Input: part model. Units: mm. Frame: model coordinates. Give positions to 0.01 mm unless a question says otherwise; leave off trailing zeros. Order: outer loops, then holes, each group sorted by start corner. A loop starts at its lowest first (then second) coordinate and runs counter-clockwise, first axis right, second up. Notation, with made-up numbers: (78.5, 39.5) -> (118.5, 39.5) arc R23 ccw to (118.5, 64.5) -> close; hole circle Ø5 at (82, 85). An arc over 180 degrees is marked (long way). Use a Markdown table: item, result. Add a question column.
from build123d import *

# Parameters (mm, degrees)
SKETCH3_R           = 12.7
SKETCH4_R           = 12.7
BOSS_EXTRUDE3_DEPTH = 330.2
SKETCH5_R           = 12.7
BOSS_EXTRUDE4_DEPTH = 330.2
SKETCH7_W           = 12.7
SKETCH7_H           = 152.4
CUT_EXTRUDE2_DEPTH  = 6.35


with BuildPart() as part:
    # Sweep1: sweep along a path in Sketch2
    with BuildLine(Plane(origin=(0, 0, 0), x_dir=(0, 0, -1), z_dir=(1, 0, 0))) as sweep1_path:
        ThreePointArc((-64.833774642, 0), (-45.844401699, 45.844401699), (0, 64.833774642))
    # Sketch3 → Sweep1 (sweep)
    with BuildSketch(Plane(origin=(0, 0, 0), x_dir=(1, 0, 0), z_dir=(0, 1, 0))):
        with Locations((0, -64.833774642)):
            Circle(SKETCH3_R)
    sweep(path=sweep1_path.line)

    # Sketch4 → Boss-Extrude3 (add)
    with BuildSketch(Plane(origin=(0, 0, 0), x_dir=(-1, 0, 0), z_dir=(0, -1, 0))):
        with Locations(Location((0, -64.833774642, 0), (0, 0, 90))):
            Circle(SKETCH4_R)
    extrude(amount=BOSS_EXTRUDE3_DEPTH)

    # Sketch5 → Boss-Extrude4 (add)
    with BuildSketch(Plane(origin=(0, 0, 0), x_dir=(-1, 0, 0), z_dir=(0, 0, -1))):
        with Locations(Location((0, 64.833774642, 0), (0, 0, 90))):
            Circle(SKETCH5_R)
    extrude(amount=BOSS_EXTRUDE4_DEPTH)

    # Sketch7 → Cut-Extrude2 (cut)
    with BuildSketch(Plane(origin=(12.7, 0, 0), x_dir=(0, 0, -1), z_dir=(1, 0, 0))):
        with Locations((-63.5, -76.2)):
            Rectangle(SKETCH7_W, SKETCH7_H)
    extrude(amount=-CUT_EXTRUDE2_DEPTH, mode=Mode.SUBTRACT)


solid = part.part
Q1. First-contact query: pin 1 (6 mm diameter, centred on x = 8.5, y = -112, fed in from -Z); pin 2 (7 mm diameter, centred on x = 10.5, z = 64.5, fed in from +Y); pin 3 (12 mm diameter, centred on x = 7, z = -6, fed in from +Y). Flat tips, straight axial feed; report the tip coordinate or a pass-through.
Q2. Section query C-C (y = -99). Return loops of the section in (x, z).
Q3. Ray query, line 1 (Z direction, x = -0.25, y = -209); line 2 (Z direction, x = 9.5, y = -92); line 3 (Y direction, x = 9.25, z = -234). Return the intervals inside material, ascending.
Q4. Section query A-A (x = 0). Return loops of the section in (y, z).
Q5. Section query B-B (z = -253). Return loops of the section in (x, y), plus the area to 3 significant figures.
Q6. Draft query along Z for faces 1 (the flat face through (0, -330.2, 65)), 2 (the flat face through (0, 65, -330.2)), 3 (the flat face through (6.35, -75, 64)), 4 (the cylindrical face through (-12.398, -162.789, 67.587)). Return one class per face: +Z half, -Z half, draft (parallel to the pull), parting line (faces both ways), or undercut.
Solution:
| question | item | result |
|---|---|---|
| 1 | pin 1 | stops at z = 53.39 |
| 1 | pin 2 | stops at y = 41.59 |
| 1 | pin 3 | stops at y = 77.49 |
| 2 | outline | (6.35, 57.15) -> (6.35, 69.85) -> (11.67, 69.85) arc R12.7 ccw (long way) to (10.11, 57.15) -> close |
| 3 | line 1 | z = 52.14 to 77.53 |
| 3 | line 2 | z = 56.41 to 57.15, 69.85 to 73.26 |
| 3 | line 3 | y = 56.13 to 73.54 |
| 4 | outline | (-330.2, 52.13) -> (0, 52.13) arc R52.13 cw to (52.13, 0) -> (52.13, -330.2) -> (77.53, -330.2) -> (77.53, 0) arc R77.53 ccw to (0, 77.53) -> (-330.2, 77.53) -> close |
| 5 | outline | circle Ø25.4 at (0, 64.83) |
| 5 | area | 507 mm² |
| 6 | face 1 | draft |
| 6 | face 2 | -Z half |
| 6 | face 3 | undercut |
| 6 | face 4 | parting line |
